Design review of the part built by this model. Coordinates are the model's own, in mm. A direction names the side the tool comes from. Round coordinates to 2 decimals unless told otherwise and drop trailing zeros. Loops run counter-clockwise (first coordinate to the right, second up) from the corner with the lowest first, then second, coordinate; pieces in that order, holes last. Notation, with made-up numbers: (66, 22.5) -> (81, 22.5) arc R26 cw to (81, 49.5) -> close; hole circle Ø1 at (-35, -0.75). An arc over 180 degrees is marked (long way). Answer as CSV lines item,"result". Start each with the question number.
(1) To check wall thickness, follow line 1 (X direction, y = 54.5, z = 1.1); line 2 (X direction, y = 21, z = 0.55); line 3 (X direction, y = 65.5, z = 2.25) (3 decimals). State the ranges of each line that lie inside material, in increasing order. Write a range as from..to.
(2) Take a section at C-C, the plane y = 21. State how many separate pieces and enclosed holes the cut face has, and give its area (3 significant figures).
(3) Take a section at D-D, the plane y = 72. Write out the cut boundary in (x, z).
(4) Draft analysis for pull direction X (two halves, no side actions). For faces 4 (the face through (31, 11.2, 1)), 5 (the face through (-33.55, 63, 1)), 6 (the face through (-27, 1, 2)), 7 (the face through (29, 36, 1)), state which applies: +X half, -X half, draft (parallel to the pull), parting line (faces both ways), or undercut.
(5) For P1, Ø1.5, axis at x = -32, z = 1.5, coming from the +Y side; P2, Ø5, axis at x = 5, y = 21.5, coming from the +Z side; P3, Ø0.9, axis at x = -31, z = 1.5, coming from the -Y side; P4, Ø1.5, axis at y = 42, z = 2, coming from the +X side, all flat-tipped, find the tip position at first contact; note any pin that passes through.
(6) Machinability: for faces 1 (the face through (-31, 11.2, 1)), 2 (the face through (0, 3, 2)), 3 (the face through (31, 61.8, 1)), which of the approach directions +Z, -Z, +X, -X, +Y, -Y give a long, thin tool a straight path to every point of the face, cutting with its end or side? Answer none if there is none.
(7) Take a section at A-A, the plane x = -3.5. Write out the cut boundary in (y, z).
(8) Take a section at B-B, the plane y = 45. Write out the cut boundary in (x, z).
from build123d import *

# Parameters (mm, degrees)
BOSS_EXTRUDE1_DEPTH = 3
SKETCH4_W           = 54
SKETCH4_H           = 3
CUT_EXTRUDE1_DEPTH  = 10


with BuildPart() as part:
    # Sketch2 → Boss-Extrude1 (new body)
    with BuildSketch(Plane.XY):
        with BuildLine():
            Line((-33.55, 0), (33.55, 0))
            Line((33.55, 0), (33.55, 11.2))
            Line((33.55, 11.2), (29, 11.2))
            Line((29, 11.2), (29, 61.8))
            Line((29, 61.8), (33.55, 61.8))
            Line((33.55, 61.8), (33.55, 64.8))
            ThreePointArc((33.55, 64.8), (0, 89.8), (-33.55, 64.8))
            Line((-33.55, 64.8), (-33.55, 61.8))
            Line((-33.55, 61.8), (-29, 61.8))
            Line((-29, 61.8), (-29, 11.2))
            Line((-29, 11.2), (-33.55, 11.2))
            Line((-33.55, 11.2), (-33.55, 0))
        make_face()
        with BuildLine():
            Line((-25.05, 64.8), (-25.05, 22.2))
            add(Edge.make_bspline(
                [(-25.05, 22.2), (-22.25, 11), (-19.45, 22.2)],
                knots=[0, 0, 0, 1, 1, 1], degree=2))
            ThreePointArc((-19.45, 22.2), (0, 16.75), (19.45, 22.2))
            add(Edge.make_bspline(
                [(19.45, 22.2), (22.25, 11), (25.05, 22.2)],
                knots=[0, 0, 0, 1, 1, 1], degree=2))
            Line((25.05, 22.2), (25.05, 64.8))
            add(Edge.make_bspline(
                [(19.632941567, 64.8), (22.187059742, 77.400349627), (25.05, 64.8)],
                knots=[0, 0, 0, 1, 1, 1], degree=2))
            ThreePointArc((19.632941567, 64.8), (0, 69.3), (-19.632941567, 64.8))
            add(Edge.make_bspline(
                [(-25.05, 64.8), (-22.187059742, 77.400349627), (-19.632941567, 64.8)],
                knots=[0, 0, 0, 1, 1, 1], degree=2))
        make_face(mode=Mode.SUBTRACT)
    extrude(amount=BOSS_EXTRUDE1_DEPTH)

    # Sketch4 → Cut-Extrude1 (cut)
    with BuildSketch(Plane.XY.offset(3)):
        with Locations((0, 1.5)):
            Rectangle(SKETCH4_W, SKETCH4_H)
    extrude(amount=-CUT_EXTRUDE1_DEPTH, mode=Mode.SUBTRACT)


solid = part.part
The answers:
1,line 1,"-29..-25.05, 25.05..29"
1,line 2,"-29..-24.73, -19.77..-17.32, 17.32..19.77, 24.73..29"
1,line 3,"-33.333..-24.887, -19.779..-18.115, 18.115..19.779, 24.887..33.333"
2,separate pieces,"4"
2,enclosed holes,"0"
2,area,"40.3 mm²"
3,outline,"(-30.49, 0) -> (30.49, 0) -> (30.49, 3) -> (-30.49, 3) -> close"
4,face 4,"draft"
4,face 5,"-X half"
4,face 6,"undercut"
4,face 7,"+X half"
5,P1,"y = 70.58"
5,P2,"through"
5,P3,"y = 0"
5,P4,"x = 29"
6,face 1,"+Z, -Z, -X"
6,face 2,"+Z, -Z, -Y"
6,face 3,"+Z, -Z, +X"
7,outline,"(3, 0) -> (16.91, 0) -> (16.91, 3) -> (3, 3) -> close; (69.16, 0) -> (89.62, 0) -> (89.62, 3) -> (69.16, 3) -> close"
8,outline,"(-29, 0) -> (-25.05, 0) -> (-25.05, 3) -> (-29, 3) -> close; (25.05, 0) -> (29, 0) -> (29, 3) -> (25.05, 3) -> close"
